```python
from build123d import *

# Parameters (mm, degrees)
SKETCH1_W           = 103
SKETCH1_H           = 52
BOSS_EXTRUDE1_DEPTH = 5
CUT_EXTRUDE1_DEPTH  = 10
CUT_EXTRUDE2_DEPTH  = 10


with BuildPart() as part:
    # Sketch1 → Boss-Extrude1 (new body)
    with BuildSketch(Plane.XY):
        Rectangle(SKETCH1_W, SKETCH1_H)
    extrude(amount=BOSS_EXTRUDE1_DEPTH)

    # Sketch2 → Cut-Extrude1 (cut)
    with BuildSketch(Plane.XY.offset(5)):
        Polygon((41.5, -26), (41.5, -22), (43, -22), (43, -18.8), (41.5, -18.8), (41.5, -11), (37.5, -11), (37.5, -18.8), (36, -18.8), (36, -22), (37.5, -22), (37.5, -26), align=None)
        Polygon((37.5, 26), (41.5, 26), (41.5, 22), (43, 22), (43, 18.8), (41.5, 18.8), (41.5, 11), (37.5, 11), (37.5, 18.8), (36, 18.8), (36, 22), (37.5, 22), align=None)
        Polygon((-37.5, -26), (-41.5, -26), (-41.5, -22), (-43, -22), (-43, -18.8), (-41.5, -18.8), (-41.5, -11), (-37.5, -11), (-37.5, -18.8), (-36, -18.8), (-36, -22), (-37.5, -22), align=None)
        Polygon((-41.5, 26), (-41.5, 22), (-43, 22), (-43, 18.8), (-41.5, 18.8), (-41.5, 11), (-37.5, 11), (-37.5, 18.8), (-36, 18.8), (-36, 22), (-37.5, 22), (-37.5, 26), align=None)
    extrude(amount=-CUT_EXTRUDE1_DEPTH, mode=Mode.SUBTRACT)

    # Sketch3 → Cut-Extrude2 (cut)
    with BuildSketch(Plane(origin=(0, 0, 0), x_dir=(-1, 0, 0), z_dir=(0, 0, -1))):
        with BuildLine():
            Line((-15, 5), (15, 5))
            ThreePointArc((15, 5), (20, 0), (15, -5))
            Line((15, -5), (-15, -5))
            ThreePointArc((-15, -5), (-20, 0), (-15, 5))
        make_face()
    extrude(amount=-CUT_EXTRUDE2_DEPTH, mode=Mode.SUBTRACT)


solid = part.part
```
Read the model definition and answer for the solid it produces. Units are mm, in the model's axes. A direction names the side the tool comes from. Give positions to 0.01 mm unless a question says otherwise; leave off trailing zeros. Write each loop counter-clockwise with the first axis right and the second up, starting at its lowest first coordinate (ties: lowest second). Pieces come first, ordered by that corner, then holes. Notation, with made-up numbers: M 19.5,33 L 58.5,33 A20 cw 58.5,48 Z; hole C -37,53.5 d6. An arc over 180 degrees is marked long. Put each result on its own line as item: value. Start each with the question number.
1. For a pull along Y with two mould halves and no side action, classify faces 5 (the flat face through (40, 11, 3)), 6 (the flat face through (-1, 6, 5)), 7 (the flat face through (-43, 20, 3)) as released by +Y, released by -Y, zero draft, split by the parting line, or undercut.
2. The part is cut by section A-A, the plane y = 13. Give the vertices of the cut face in (x, z), and give its area (3 significant figures).
3. The part is cut by section C-C, the plane y = -4. Give the vertices of the cut face in (x, z), and give its area (3 significant figures).
4. Which of the six approach directions +Z, -Z, +X, -X, +Y, -Y give full straight-line access (tool end or side, diameter ignored) to faces 1 (the flat face through (51.5, 0, 2)), 2 (the flat face through (-40, -11, 3)), 3 (the flat face through (37.5, 15, 3)), 4 (the flat face through (43, 20, 3))?
5. Consider line 1 along X through (y, z) = (19, 0.35); line 2 along X through (y, z) = (13.5, 1.45); line 3 along Y through (x, z) = (-12.5, 1.6). Determine where each line is inside the solid, lowest interval first.
6. The part is cut by section B-B, the plane x = -12. Give the vertices of the cut face in (y, z), and give its area (3 significant figures).
Final values:
1. face 5: released by +Y
1. face 6: zero draft
1. face 7: undercut
2. outline: M -51.5,0 L -41.5,0 L -41.5,5 L -51.5,5 Z; M -37.5,0 L 37.5,0 L 37.5,5 L -37.5,5 Z; M 41.5,0 L 51.5,0 L 51.5,5 L 41.5,5 Z
2. area: 475 mm²
3. outline: M -51.5,0 L -18,0 L -18,5 L -51.5,5 Z; M 18,0 L 51.5,0 L 51.5,5 L 18,5 Z
3. area: 335 mm²
4. face 1: +Z, -Z, +X, +Y, -Y
4. face 2: +Z, -Z, -Y
4. face 3: +Z, -Z, +Y
4. face 4: +Z, -Z
5. line 1: x = -51.5 to -43, -36 to 36, 43 to 51.5
5. line 2: x = -51.5 to -41.5, -37.5 to 37.5, 41.5 to 51.5
5. line 3: y = -26 to -5, 5 to 26
6. outline: M -26,0 L -5,0 L -5,5 L -26,5 Z; M 5,0 L 26,0 L 26,5 L 5,5 Z
6. area: 210 mm²
